Verification items for the finished model (mm, model axes). A direction names the side the tool comes from. Give positions to 0.01 mm unless a question says otherwise; leave off trailing zeros. Order: outer loops, then holes, each group sorted by start corner. A loop starts at its lowest first (then second) coordinate and runs counter-clockwise, first axis right, second up.
from build123d import *

# Parameters (mm, degrees)
F0_R      = 5
F1_DEPTH  = 2
F2_DEPTH  = 15
F3_W      = 5
F3_H      = 15
F4_DEPTH  = 10
F5_SIZE   = 4
F6_W      = 7
F6_H      = 7
F7_DEPTH  = 4.5
F8_W      = 5
F8_H      = 15
F9_DEPTH  = 10
F10_W     = 7
F10_H     = 7
F11_DEPTH = 4.5
F12_SIZE  = 4


with BuildPart() as f1:
    # F0 (on Top) → F1 (new body)
    with BuildSketch(Plane.XY):
        Polygon((25.5, 17.5), (25.5, 25.5), (-25.5, 25.5), (-25.5, -25.5), (-17.5, -25.5), (-15, -25.5), (25.5, -25.5), (25.5, 15), align=None)
        Circle(F0_R, mode=Mode.SUBTRACT)
    extrude(amount=F1_DEPTH)

    # F0 (on Top) → F2 (join)
    with BuildSketch(Plane.XY):
        Polygon((25.5, 27.5), (-27.5, 27.5), (-27.5, -25.5), (-25.5, -25.5), (-25.5, 25.5), (25.5, 25.5), align=None)
        Polygon((27.5, -27.5), (27.5, 15), (25.5, 15), (25.5, -25.5), (-15, -25.5), (-15, -27.5), align=None)
    extrude(amount=F2_DEPTH)

    # F3 (on face) → F4 (join)
    with BuildSketch(Plane.XZ.offset(27.5)):
        with Locations((-12.5, 7.5)):
            Rectangle(F3_W, F3_H)
    extrude(amount=F4_DEPTH)

    # F5
    f5_edges = [f1.edges().sort_by_distance(p)[0] for p in [
        (-12.5, -37.5, 15),
        (-12.5, -37.5, 0),
    ]]
    chamfer(f5_edges, length=F5_SIZE)

    # F6 (on face) → F7 (cut)
    with BuildSketch(Plane.YZ.offset(-10)):
        with Locations((-32, 7.5)):
            Rectangle(F6_W, F6_H)
    extrude(amount=-F7_DEPTH, mode=Mode.SUBTRACT)

    # F8 (on face) → F9 (join)
    with BuildSketch(Plane.YZ.offset(27.5)):
        with Locations((12.5, 7.5)):
            Rectangle(F8_W, F8_H)
    extrude(amount=F9_DEPTH)

    # F10 (on face) → F11 (cut)
    with BuildSketch(Plane.XZ.offset(-10)):
        with Locations((32, 7.5)):
            Rectangle(F10_W, F10_H)
    extrude(amount=-F11_DEPTH, mode=Mode.SUBTRACT)

    # F12
    f12_edges = [f1.edges().sort_by_distance(p)[0] for p in [
        (37.5, 12.5, 15),
        (37.5, 12.5, 0),
    ]]
    chamfer(f12_edges, length=F12_SIZE)


solid = f1.part
(1) Set-up check for faces 1 (the flat face through (35.5, 12, 7)), 2 (the flat face through (-15, -31, 7)), 3 (the flat face through (25.5, 26, 4)), 4 (the flat face through (8, -27.5, 7)), 5 (the flat face through (-25.5, 0, 8)): record each of +Z, -Z, +X, -X, +Y, -Y from which the full face is reachable in a straight line by a thin tool's end or side.
Solved:
face 1: -Y
face 2: +Z, -Z, -X, -Y
face 3: +Z, -Z, +X, +Y
face 4: +Z, -Z, +X, -Y
face 5: +Z, -Y
(2) Release check for a two-part mould opening along X. For faces 6 (the flat face through (28.5, 12, 7)), 7 (the flat face through (-13, 27, 15)), 8 (the flat face through (-27.5, 1, 7)), 9 (the flat face through (37.5, 12, 8)) record: pulls with the +X half, pulls with the -X half, needs draft (parallel to the pull), parting line crosses it, or undercut.
Solved:
face 6: undercut
face 7: needs draft
face 8: pulls with the -X half
face 9: pulls with the +X half
(3) Scan lines: line 1 (Y direction, x = 0, z = 1.55); line 2 (Y direction, x = -5.5, z = 4.5); line 3 (Y direction, x = -11.5, z = 5.75). Record each from-to range of solid material in increasing order.
Solved:
line 1: y = -27.5 to -5, 5 to 27.5
line 2: y = -27.5 to -25.5, 25.5 to 27.5
line 3: y = -37.5 to -35.5, -28.5 to -25.5, 25.5 to 27.5
(4) Section check A-A, the plane x = 0. Enter the section's corners in (y, z).
Solved:
outline: (-27.5, 0) - (-5, 0) - (-5, 2) - (-25.5, 2) - (-25.5, 15) - (-27.5, 15) - close; (5, 0) - (27.5, 0) - (27.5, 15) - (25.5, 15) - (25.5, 2) - (5, 2) - close
(5) Go/stop test with flat-tipped pins: pin 1 (3 mm diameter, centred on y = 0, z = 6.5, fed in from +X); pin 2 (5.5 mm diameter, centred on x = 33, z = 8.5, fed in from -Y); pin 3 (6 mm diameter, centred on x = 33.5, z = 5.5, fed in from +Y). Record where each tip stops, or that it passes through.
Solved:
pin 1: stops at x = 27.5
pin 2: stops at y = 10
pin 3: stops at y = 15
(6) Section check C-C, the plane z = 6. Enter the section's corners in (x, y), then the cut area to 3 significant figures.
Solved:
outline: (-27.5, -25.5) - (-25.5, -25.5) - (-25.5, 25.5) - (25.5, 25.5) - (25.5, 27.5) - (-27.5, 27.5) - close; (-15, -37.5) - (-10, -37.5) - (-10, -35.5) - (-14.5, -35.5) - (-14.5, -28.5) - (-10, -28.5) - (-10, -27.5) - (27.5, -27.5) - (27.5, 10) - (28.5, 10) - (28.5, 14.5) - (35.5, 14.5) - (35.5, 10) - (37.5, 10) - (37.5, 15) - (25.5, 15) - (25.5, -25.5) - (-15, -25.5) - close
area: 411 mm2
(7) Section check B-B, the plane z = 1.25. Enter the section's corners in (x, y).
Solved:
outline: (-27.5, -25.5) - (-15, -25.5) - (-15, -34.75) - (-10, -34.75) - (-10, -27.5) - (27.5, -27.5) - (27.5, 10) - (34.75, 10) - (34.75, 15) - (25.5, 15) - (25.5, 27.5) - (-27.5, 27.5) - close; hole circle Ø10 at (0, 0)
